```python
from build123d import *

# Parameters (mm, degrees)
SKETCH1_W           = 381
SKETCH1_H           = 177.8
BOSS_EXTRUDE1_DEPTH = 3.175
CUT_EXTRUDE1_DEPTH  = 211.246380766
CUT_EXTRUDE2_DEPTH  = 205.829884405
CUT_EXTRUDE3_DEPTH  = 200.326767223
SKETCH9_R           = 2.413
CUT_EXTRUDE5_DEPTH  = 200.326767223
CUT_EXTRUDE6_DEPTH  = 200.326767223
CUT_EXTRUDE7_DEPTH  = 190.367896253
SKETCH12_R          = 2.413
CUT_EXTRUDE8_DEPTH  = 188.550586603


with BuildPart() as part:
    # Sketch1 → Boss-Extrude1 (new body)
    with BuildSketch(Plane.XY):
        Rectangle(SKETCH1_W, SKETCH1_H)
    extrude(amount=BOSS_EXTRUDE1_DEPTH)

    # Sketch3 → Cut-Extrude1 (cut, through all)
    with BuildSketch(Plane(origin=(0, 0, 0), x_dir=(-1, 0, 0), z_dir=(0, 0, -1))):
        Polygon((-190.5, 88.9), (-139.670694847, 88.9), (-190.5, -121.745827518), align=None)
        Polygon((190.5, 88.9), (141.601183723, 88.9), (190.5, -113.745532698), align=None)
    extrude(amount=-CUT_EXTRUDE1_DEPTH, mode=Mode.SUBTRACT)

    # Sketch4 → Cut-Extrude2 (cut, through all)
    with BuildSketch(Plane(origin=(0, 0, 0), x_dir=(-1, 0, 0), z_dir=(0, 0, -1))):
        Polygon((178.375641573, -63.5), (-176.445152697, -63.5), (-182.574229005, -88.9), (184.504717881, -88.9), align=None)
    extrude(amount=-CUT_EXTRUDE2_DEPTH, mode=Mode.SUBTRACT)

    # Sketch8 → Cut-Extrude3 (cut, through all)
    with BuildSketch(Plane(origin=(0, 0, 0), x_dir=(-1, 0, 0), z_dir=(0, 0, -1))):
        Polygon((-139.864527638, -63.5), (-127.945162942, -14.118133437), (132.284027695, -14.118133437), (144.203392391, -63.5), align=None)
    extrude(amount=-CUT_EXTRUDE3_DEPTH, mode=Mode.SUBTRACT)

    # Sketch9 → Cut-Extrude5 (cut, through all)
    with BuildSketch(Plane(origin=(0, 0, 0), x_dir=(-1, 0, 0), z_dir=(0, 0, -1))):
        with Locations((-152.192493977, -47.625)):
            Circle(SKETCH9_R)
        with Locations((-149.151314542, -35.414265987)):
            Circle(SKETCH9_R)
        with Locations((-146.110135107, -23.203531973)):
            Circle(SKETCH9_R)
        with Locations((-143.068955672, -10.99279796)):
            Circle(SKETCH9_R)
        with Locations((-140.027776237, 1.217936053)):
            Circle(SKETCH9_R)
        with Locations((-136.986596801, 13.428670067)):
            Circle(SKETCH9_R)
        with Locations((-133.945417366, 25.63940408)):
            Circle(SKETCH9_R)
        with Locations((-124.821879061, 62.27160612)):
            Circle(SKETCH9_R)
        with Locations((-121.780699626, 74.482340133)):
            Circle(SKETCH9_R)
    extrude(amount=-CUT_EXTRUDE5_DEPTH, mode=Mode.SUBTRACT)

    # Sketch10 → Cut-Extrude6 (cut, through all)
    with BuildSketch(Plane(origin=(0, 0, 0), x_dir=(-1, 0, 0), z_dir=(0, 0, -1))):
        Polygon((-139.670694847, 88.9), (-151.928847464, 38.1), (153.859336339, 38.1), (141.601183723, 88.9), align=None)
    extrude(amount=-CUT_EXTRUDE6_DEPTH, mode=Mode.SUBTRACT)

    # Sketch11 → Cut-Extrude7 (cut, through all)
    with BuildSketch(Plane(origin=(0, 0, 0), x_dir=(-1, 0, 0), z_dir=(0, 0, -1))):
        Polygon((-127.945162942, -14.118133437), (-56.620358568, 12.7), (-56.620358568, 38.1), (60.959223321, 38.1), (153.859336339, 38.1), (178.375641573, -63.5), (144.203392391, -63.5), (132.284027695, -14.118133437), align=None)
    extrude(amount=-CUT_EXTRUDE7_DEPTH, mode=Mode.SUBTRACT)

    # Sketch12 → Cut-Extrude8 (cut, through all)
    with BuildSketch(Plane(origin=(0, 0, 0), x_dir=(-1, 0, 0), z_dir=(0, 0, -1))):
        with Locations((-62.970358568, 25.4)):
            Circle(SKETCH12_R)
        with Locations((-75.670358568, 25.4)):
            Circle(SKETCH12_R)
        with Locations((-88.370358568, 25.4)):
            Circle(SKETCH12_R)
    extrude(amount=-CUT_EXTRUDE8_DEPTH, mode=Mode.SUBTRACT)


solid = part.part
```
Geometry check sheet. Reference: the model listing, model coordinates, mm. Coordinates: 2 decimals unless noted, no trailing zeros. Order: outer loops, then holes, each group sorted by start corner. A loop starts at its lowest first (then second) coordinate and runs counter-clockwise, first axis right, second up. Notation, with made-up numbers: (45, -14) - (52, -14) arc R18 cw to (52, 12) - close; hole circle Ø2 at (41.25, 83.25). An arc over 180 degrees is marked (long way). Answer in a Markdown table with one row per item. Add a question column.
1. Material ranges on L1, parallel to Y at x = 146, z = 3.05; L2, parallel to X at y = -24, z = 2.75; L3, parallel to Y at x = 88.5, z = 2.6, recorded low to high. Write a range as [from, to].
2. Section check D-D (x = 167). Enter the section's corners in (y, z) (3 decimals).
3. Section check C-C (x = 89). Enter the section's corners in (y, z) (3 decimals).
4. Gauge pin test, flat ends, axial feed: pin 1 Ø4.5 at (x, y) = (133.95, 25.64) entering from -Z; pin 2 Ø1.5 at (y, z) = (-7.5, 2.5) entering from +X; pin 3 Ø1 at (y, z) = (9.5, 0.5) entering from +X. Record the tip position at first contact, or that the pin passes through.
5. Section check A-A (x = 64). Enter the section's corners in (y, z) (3 decimals), plus the area to 3 significant figures.
6. Section check B-B (z = 1.25). Give the number of separate pieces and of enclosed holes in the cut face, plus the area to 3 significant figures.
7. Draft check along Y on faces 1 (the face through (143.8, -22.5, 1.6)), 2 (the face through (158, -63.5, 2)), 3 (the face through (129, -1, 0)). Enter one of: +Y half, -Y half, draft (parallel to the pull), parting line (faces both ways), or undercut.
Data:
| question | item | result |
|---|---|---|
| 1 | L1 | y = [-63.5, -25.61], [-20.79, 38.1] |
| 1 | L2 | x = [130.33, 143.83], [148.39, 166.91] |
| 1 | L3 | y = [0.71, 22.99], [27.81, 38.1] |
| 2 | outline | (-63.5, 0) - (-24.358, 0) - (-24.358, 3.175) - (-63.5, 3.175) - close |
| 3 | outline | (0.525, 0) - (23.071, 0) - (23.071, 3.175) - (0.525, 3.175) - close; (27.729, 0) - (38.1, 0) - (38.1, 3.175) - (27.729, 3.175) - close |
| 4 | pin 1 | passes through |
| 4 | pin 2 | stops at x = 163.11 |
| 4 | pin 3 | stops at x = 158.95 |
| 5 | outline | (9.925, 0) - (23.218, 0) - (23.218, 3.175) - (9.925, 3.175) - close; (27.582, 0) - (38.1, 0) - (38.1, 3.175) - (27.582, 3.175) - close |
| 5 | area | 75.6 mm² |
| 6 | separate pieces | 1 |
| 6 | enclosed holes | 10 |
| 6 | area | 5,970 mm² |
| 7 | face 1 | undercut |
| 7 | face 2 | -Y half |
| 7 | face 3 | draft |
